For this review, take the finished solid that the model builds, in its own axes (mm). A direction names the side the tool comes from. Round coordinates to 2 decimals unless told otherwise and drop trailing zeros. Order: outer loops, then holes, each group sorted by start corner. A loop starts at its lowest first (then second) coordinate and runs counter-clockwise, first axis right, second up. Notation, with made-up numbers: M -22,61.25 L -18,61.25 A18 cw -18,71.25 Z; hole C 22.5,-4.75 d11. An arc over 180 degrees is marked long. Answer in a Markdown table with one row per item. Add a question column.
```python
from build123d import *

# Parameters (mm, degrees)
SKETCH1_W           = 80
SKETCH1_H           = 80
BOSS_EXTRUDE1_DEPTH = 30
SHELL1_T            = -5
SKETCH3_R           = 10
CUT_EXTRUDE1_DEPTH  = 10


with BuildPart() as part:
    # Sketch1 → Boss-Extrude1 (new body)
    with BuildSketch(Plane.XY):
        Rectangle(SKETCH1_W, SKETCH1_H)
    extrude(amount=BOSS_EXTRUDE1_DEPTH)

    # Shell1
    shell1_openings = [part.faces().sort_by_distance(p)[0] for p in [
        (0, 0, 0),
    ]]
    offset(amount=SHELL1_T, openings=shell1_openings, kind=Kind.INTERSECTION)

    # Sketch3 → Cut-Extrude1 (cut)
    with BuildSketch(Plane.XY.offset(30)):
        Circle(SKETCH3_R)
    extrude(amount=-CUT_EXTRUDE1_DEPTH, mode=Mode.SUBTRACT)


solid = part.part
```
1. For faces 1 (the flat face through (-36, 0, 0)), 2 (the flat face through (-35, 0, 12)), list the 3-axis set-ups (+Z, -Z, +X, -X, +Y, -Y) from which the entire face can be reached by the end or side of a thin tool; tool diameter is ignored.
2. Clearance check with a flat-ended pin moving along its axis: pin 1 Ø5 at (x, y) = (15.5, 11.5) entering from -Z. State where the tip first meets the part, or that it passes through.
3. To check wall thickness, follow probe 1 along X at (y, z) = (30.5, 2.25); probe 2 along Y at (x, z) = (0, 27.9). State the ranges of each line that lie inside material, in increasing order. Write a range as [from, to].
4. The part is to be moulded in two halves that separate along X. For faces 3 (the flat face through (35, 0, 12)), 4 (the flat face through (-40, -1, 15)), 5 (the flat face through (0, 35, 12)), 6 (the flat face through (-1, -40, 15)), say which applies: pulls with the +X half, pulls with the -X half, needs draft (parallel to the pull), parting line crosses it, or undercut.
5. Consider section A-A on x = 0. Write out the cut boundary in (y, z), plus the area to 3 significant figures.
6. Consider section B-B on z = 8.75. Write out the cut boundary in (x, y), plus the area to 3 significant figures.
7. Consider section D-D on x = -33. Write out the cut boundary in (y, z), plus the area to 3 significant figures.
Solved:
| question | item | result |
|---|---|---|
| 1 | face 1 | -Z, +X, -X, +Y, -Y |
| 1 | face 2 | -Z |
| 2 | pin 1 | stops at z = 25 |
| 3 | probe 1 | x = [-40, -35], [35, 40] |
| 3 | probe 2 | y = [-40, -10], [10, 40] |
| 4 | face 3 | undercut |
| 4 | face 4 | pulls with the -X half |
| 4 | face 5 | undercut |
| 4 | face 6 | needs draft |
| 5 | outline | M -40,0 L -35,0 L -35,25 L -10,25 L -10,30 L -40,30 Z; M 10,25 L 35,25 L 35,0 L 40,0 L 40,30 L 10,30 Z |
| 5 | area | 550 mm^2 |
| 6 | outline | M -40,-40 L 40,-40 L 40,40 L -40,40 Z; hole M -35,-35 L 35,-35 L 35,35 L -35,35 Z |
| 6 | area | 1,500 mm^2 |
| 7 | outline | M -40,0 L -35,0 L -35,25 L 35,25 L 35,0 L 40,0 L 40,30 L -40,30 Z |
| 7 | area | 650 mm^2 |
